Here's how the part is built. I have some questions about the finished solid (model axes, mm). Give positions to 0.01 mm unless a question says otherwise; leave off trailing zeros. Order: outer loops, then holes, each group sorted by start corner. A loop starts at its lowest first (then second) coordinate and runs counter-clockwise, first axis right, second up. Notation, with made-up numbers: M 67.25,12.25 L 79.25,12.25 A17 ccw 79.25,30.25 Z; hole C 71.25,6.25 d10. An arc over 180 degrees is marked long. Use one line per item in the form item = value.
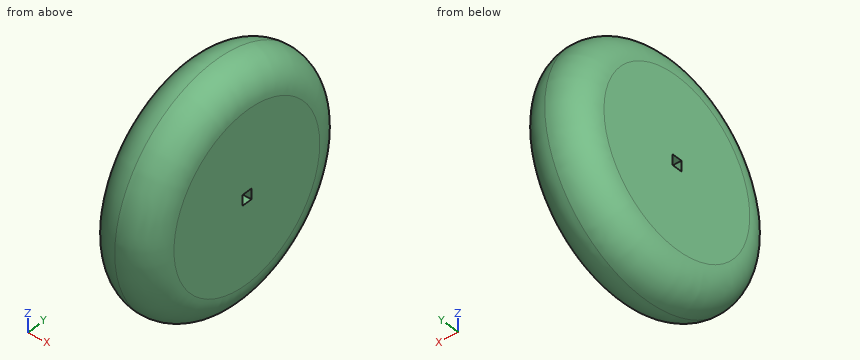
from build123d import *

# Parameters (mm, degrees)
F2_W     = 3.175
F2_H     = 3.175
F3_DEPTH = 25


with BuildPart() as f1:
    # F0 (on Top) → F1 (revolve)
    with BuildSketch(Plane.XY):
        with BuildLine():
            Line((-9.525, 0), (9.525, 0))
            Line((9.525, 0), (9.525, 25.4))
            ThreePointArc((9.525, 25.4), (6.735192, 32.135192), (0, 34.925))
            ThreePointArc((0, 34.925), (-6.735192, 32.135192), (-9.525, 25.4))
            Line((-9.525, 25.4), (-9.525, 0))
        make_face()
    revolve(axis=Axis((0, 0, 0), (-1, 0, 0)))

    # F2 (on face) → F3 (cut)
    with BuildSketch(Plane.YZ.offset(9.525)):
        Rectangle(F2_W, F2_H)
    extrude(amount=-F3_DEPTH, mode=Mode.SUBTRACT)


solid = f1.part
Q1. I want a section at B-B on x = 6.5. Write out the boundary of the cut face in (y, z), then the cut area to 3 significant figures.
Found:
outline = C 0,0 d64.72; hole M -1.59,-1.59 L 1.59,-1.59 L 1.59,1.59 L -1.59,1.59 Z
area = 3,280 mm²
Q2. I need wall thicknesses on L1, parallel to X at y = -25, z = -6; L2, parallel to Y at x = 3.25, z = 4; L3, parallel to Z at x = 5.75, y = -20. Which ranges of each line are inside material? Lowest first, please.
Found:
L1 = -9.52 to 9.52
L2 = -34.12 to 34.12
L3 = -26.24 to 26.24
Q3. I want a section at A-A on x = 2.5. Write out the boundary of the cut face in (y, z).
Found:
outline = C 0,0 d69.18; hole M -1.59,-1.59 L 1.59,-1.59 L 1.59,1.59 L -1.59,1.59 Z
Q4. I'm going to push flat-ended pins straight in: pin 1 Ø3.5 at (x, z) = (-4, 0) entering from +Y; pin 2 Ø4 at (x, z) = (6, -12.5) entering from +Y; pin 3 Ø1.6 at (x, z) = (-4, 0.5) entering from -Y. Where does each tip first touch, or does it pass through?
Found:
pin_1 = 34.66
pin_2 = 31.91
pin_3 = -34.37
